Print and shaded views of the part. All mm, measured from the part's lowest x, y and z. Round coordinates to 2 decimals unless told otherwise and drop trailing zeros. Order: outer loops, then holes, each group sorted by start corner. A loop starts at its lowest first (then second) coordinate and runs counter-clockwise, first axis right, second up. Notation, with made-up numbers: (-4, 37.5) - (0, 37.5) arc R20 cw to (0, 61.5) - close; hole circle Ø5 at (63.5, 33.5). An arc over 180 degrees is marked (long way). Write item = value, one per line.
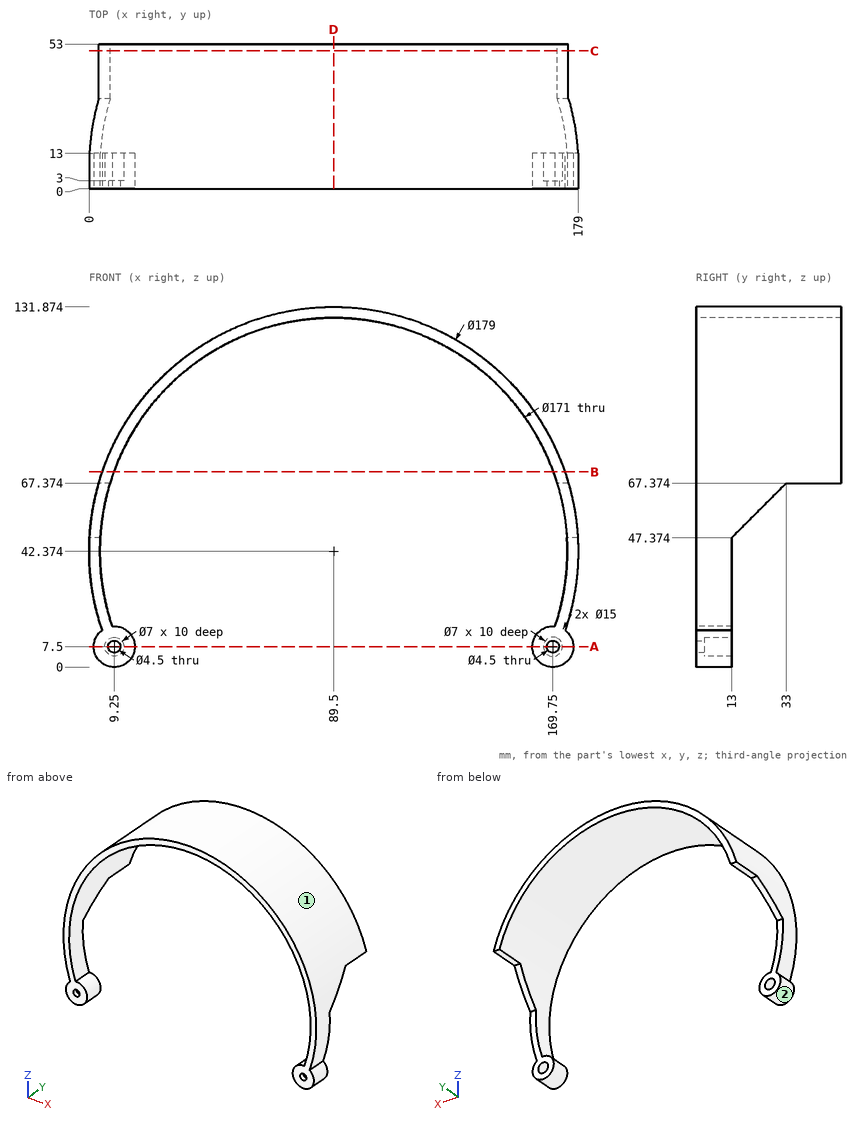
(1) Band-saw the part on B-B on z = 71.5. List the corners of the cut face in (x, y), plus the area to 3 significant figures.
Solved:
outline = (4.87, 0) - (9.11, 0) - (9.11, 53) - (4.87, 53) - close; (169.89, 0) - (174.13, 0) - (174.13, 53) - (169.89, 53) - close
area = 450 mm²
(2) Probe line 1 along X through (y, z) = (0.6, 7.5); line 2 along X through (y, z) = (42.5, 86); line 3 along X through (y, z) = (19.5, 89) (1 decimal). List the from-to ranges inside material, lowest first.
Solved:
line_1 = 1.75 to 7, 11.5 to 16.75, 162.25 to 167.5, 172 to 177.25
line_2 = 11.35 to 15.97, 163.03 to 167.65
line_3 = 13.1 to 17.8, 161.2 to 165.9
(3) Band-saw the part on C-C on y = 50.5. List the corners of the cut face in (x, z).
Solved:
outline = (3.56, 67.37) - (7.74, 67.37) arc R85.5 cw to (171.26, 67.37) - (175.44, 67.37) arc R89.5 ccw to start
(4) Band-saw the part on A-A on z = 7.5. List the corners of the cut face in (x, y), plus the area to 3 significant figures.
Solved:
outline = (1.75, 0) - (7, 0) - (7, 3) - (5.75, 3) - (5.75, 13) - (1.75, 13) - close; (11.5, 0) - (16.75, 0) - (16.75, 13) - (12.75, 13) - (12.75, 3) - (11.5, 3) - close; (162.25, 0) - (167.5, 0) - (167.5, 3) - (166.25, 3) - (166.25, 13) - (162.25, 13) - close; (172, 0) - (177.25, 0) - (177.25, 13) - (173.25, 13) - (173.25, 3) - (172, 3) - close
area = 223 mm²
(5) Pull direction X, two halves, no side cores. Call the marked faces 1 and 2: released by +X, released by -X, zero draft, split by the parting line, or undercut.
Solved:
face_1 = split by the parting line
face_2 = undercut
(6) Drop flat-ended pins along their axis: pin 1 (8 mm diameter, centred on x = 97.5, y = 40, fed in from -Z); pin 2 (3 mm diameter, centred on x = 51, y = 28.5, fed in from +Z); pin 3 (3.5 mm diameter, centred on x = 170.5, z = 8.5, fed in from +Y); pin 4 (8 mm diameter, centred on x = 9.25, z = 7.5, fed in from -Y). Give the stop position or say it passes through.
Solved:
pin_1 = 127.03
pin_2 = 123.87
pin_3 = 3
pin_4 = 0
(7) Band-saw the part on D-D on x = 89.5. List the corners of the cut face in (y, z), plus the area to 3 significant figures.
Solved:
outline = (0, 127.87) - (53, 127.87) - (53, 131.87) - (0, 131.87) - close
area = 212 mm²
